from build123d import *

# Parameters (mm, degrees)
SKETCH1_R           = 50.8
BOSS_EXTRUDE1_DEPTH = 50.8
SKETCH3_W           = 98.373776994
SKETCH3_H           = 25.4
BOSS_EXTRUDE3_DEPTH = 63.5
SKETCH4_R           = 12.7
CUT_EXTRUDE1_DEPTH  = 104.175287739
FILLET1_R           = 25.4
FILLET2_R           = 25.4
SKETCH5_W           = 25.4
SKETCH5_H           = 98.373776994
BOSS_EXTRUDE4_DEPTH = 50.8
SKETCH6_R           = 12.7
CUT_EXTRUDE2_DEPTH  = 50.8
FILLET3_R           = 25.4


with BuildPart() as part:
    # Sketch1 → Boss-Extrude1 (new body)
    with BuildSketch(Plane(origin=(0, 0, 0), x_dir=(1, 0, 0), z_dir=(0, 1, 0))):
        with Locations(Location((0, 0, 0), (0, 0, 270))):
            Circle(SKETCH1_R)
    extrude(amount=BOSS_EXTRUDE1_DEPTH)

    # Sketch3 → Boss-Extrude3 (add)
    with BuildSketch(Plane.XZ):
        Rectangle(SKETCH3_W, SKETCH3_H)
    extrude(amount=BOSS_EXTRUDE3_DEPTH)

    # Sketch4 → Cut-Extrude1 (cut, through all)
    with BuildSketch(Plane.XY.offset(12.7)):
        with Locations((0.243990196, -31.967064289)):
            Circle(SKETCH4_R)
    extrude(amount=-CUT_EXTRUDE1_DEPTH, mode=Mode.SUBTRACT)

    # Fillet1
    fillet1_edges = [part.edges().sort_by_distance(p)[0] for p in [
        (-49.186888497, -63.5, 0),
    ]]
    fillet(fillet1_edges, radius=FILLET1_R)

    # Fillet2
    fillet2_edges = [part.edges().sort_by_distance(p)[0] for p in [
        (49.186888497, -63.5, 0),
    ]]
    fillet(fillet2_edges, radius=FILLET2_R)

    # Sketch5 → Boss-Extrude4 (add)
    with BuildSketch(Plane(origin=(0, 50.8, 0), x_dir=(1, 0, 0), z_dir=(0, 1, 0))):
        Rectangle(SKETCH5_W, SKETCH5_H)
    extrude(amount=BOSS_EXTRUDE4_DEPTH)

    # Sketch6 → Cut-Extrude2 (cut)
    with BuildSketch(Plane(origin=(12.7, 0, 0), x_dir=(0, 0, -1), z_dir=(1, 0, 0))):
        with Locations((0, 76.2)):
            Circle(SKETCH6_R)
    extrude(amount=-CUT_EXTRUDE2_DEPTH, mode=Mode.SUBTRACT)

    # Fillet3
    fillet3_edges = [part.edges().sort_by_distance(p)[0] for p in [
        (0, 101.6, -49.186888497),
        (0, 101.6, 49.186888497),
    ]]
    fillet(fillet3_edges, radius=FILLET3_R)


solid = part.part
Check sheet for the modelled part. Datum: model origin and axes. Units: mm. A direction names the side the tool comes from. Round coordinates to 2 decimals unless told otherwise and drop trailing zeros. Loops run counter-clockwise (first coordinate to the right, second up) from the corner with the lowest first, then second, coordinate; pieces in that order, holes last.
1. Mould release check, pull along X, two halves, no side actions. Record for faces 1 (the flat face through (0, 101.6, 0)), 2 (the flat face through (12.7, 70, 12)), 3 (the cylindrical face through (-2.509, -44.365, 0.178)), 4 (the flat face through (-12.7, 70, 12)): released by +X, released by -X, zero draft, split by the parting line, or undercut.
2. Gauge pin test, flat ends, axial feed: pin 1 Ø8 at (x, y) = (-15.5, 68.5) entering from +Z; pin 2 Ø1.5 at (y, z) = (82, 38.5) entering from -X; pin 3 Ø8 at (y, z) = (-33, -9) entering from -X. Record the tip position at first contact, or that the pin passes through.
3. Scan lines: probe 1 along Y at (x, z) = (0.75, 0); probe 2 along Y at (x, z) = (5.5, 0); probe 3 along Y at (x, z) = (-14, -36). Record each from-to range of solid material in increasing order.
4. Sectioned sample at C-C on y = 81. Record the boundary of the cut face in (x, z), and give its area (3 significant figures).
5. Set-up check for faces 5 (the flat face through (0, 63, 49.187)), 6 (the flat face through (49.187, -19, 0)), 7 (the flat face through (1, 0, 27)), 8 (the flat face through (0, 63, -49.187)), 9 (the flat face through (-12, -24, -12.7)): record each of +Z, -Z, +X, -X, +Y, -Y from which the full face is reachable in a straight line by a thin tool's end or side.
6. Sectioned sample at D-D on z = -40. Record the boundary of the cut face in (x, y), and give its area (3 significant figures).
7. Sectioned sample at B-B on z = 6. Record the boundary of the cut face in (x, y).
8. Sectioned sample at A-A on x = 0. Record the boundary of the cut face in (y, z).
Recorded:
1. face 1: zero draft
1. face 2: released by +X
1. face 3: undercut
1. face 4: released by -X
2. pin 1: stops at z = 49.19
2. pin 2: stops at x = -12.7
2. pin 3: stops at x = -49.19
3. probe 1: y = -63.5 to -44.66, -19.28 to 63.5, 88.9 to 101.6
3. probe 2: y = -63.5 to -43.53, -20.41 to 63.5, 88.9 to 101.6
3. probe 3: y = 0 to 50.8
4. outline: (-12.7, -48.73) - (12.7, -48.73) - (12.7, -11.76) - (-12.7, -11.76) - close; (-12.7, 11.76) - (12.7, 11.76) - (12.7, 48.73) - (-12.7, 48.73) - close
4. area: 1,880 mm2
5. face 5: +Z, +X, -X, +Y
5. face 6: +Z, -Z, +X, -Y
5. face 7: +Z, +X, -X, -Y
5. face 8: -Z, +X, -X, +Y
5. face 9: -Z, +X, -X, -Y
6. outline: (-31.32, 0) - (31.32, 0) - (31.32, 50.8) - (12.7, 50.8) - (12.7, 95.75) - (-12.7, 95.75) - (-12.7, 50.8) - (-31.32, 50.8) - close
6. area: 4,320 mm2
7. outline: (-50.44, 0) - (-49.19, 0) - (-49.19, -38.1) arc R25.4 ccw to (-23.79, -63.5) - (23.79, -63.5) arc R25.4 ccw to (49.19, -38.1) - (49.19, 0) - (50.44, 0) - (50.44, 50.8) - (12.7, 50.8) - (12.7, 65.01) - (-12.7, 65.01) - (-12.7, 50.8) - (-50.44, 50.8) - close; (-12.7, 87.39) - (12.7, 87.39) - (12.7, 101.6) - (-12.7, 101.6) - close; hole circle Ø25.4 at (0.24, -31.97)
8. outline: (-63.5, -12.7) - (-44.66, -12.7) - (-44.66, 12.7) - (-63.5, 12.7) - close; (-19.27, -12.7) - (0, -12.7) - (0, -50.8) - (50.8, -50.8) - (50.8, -49.19) - (76.2, -49.19) arc R25.4 ccw to (101.6, -23.79) - (101.6, 23.79) arc R25.4 ccw to (76.2, 49.19) - (50.8, 49.19) - (50.8, 50.8) - (0, 50.8) - (0, 12.7) - (-19.27, 12.7) - close; hole circle Ø25.4 at (76.2, 0)
